from build123d import *

# Parameters (mm, degrees)
F1_DEPTH = 90
F2_R     = 10
F3_DEPTH = 300
F4_R     = 5
F5_DEPTH = 104.001


with BuildPart() as f1:
    # F0 (on Front) → F1 (new body)
    with BuildSketch(Plane.XZ):
        Polygon((50, 0), (0, 0), (-50, 0), (-50, 150), (-52, 150), (-52, -2), (52, -2), (52, 150), (50, 150), align=None)
    extrude(amount=F1_DEPTH)

    # F2 (on face) → F3 (join)
    with BuildSketch(Plane(origin=(0, 0, -2), x_dir=(1, 0, 0), z_dir=(0, 0, -1))):
        with Locations((0, 45)):
            Circle(F2_R)
    extrude(amount=F3_DEPTH)

    # F4 (on face) → F5 (cut, through all)
    with BuildSketch(Plane(origin=(-52, 0, 0), x_dir=(0, -1, 0), z_dir=(-1, 0, 0))):
        with Locations((45, 100)):
            Circle(F4_R)
        with Locations((45, 50)):
            Circle(F4_R)
    extrude(amount=-F5_DEPTH, mode=Mode.SUBTRACT)


solid = f1.part
Can you work these out from the model? Positions are in its coordinate system, mm. A direction names the side the tool comes from. Coordinates: 2 decimals unless noted, no trailing zeros. Write each loop counter-clockwise with the first axis right and the second up, starting at its lowest first coordinate (ties: lowest second). Pieces come first, ordered by that corner, then holes. Notation, with made-up numbers: (-37.75, 3.25) -> (8.25, 3.25) arc R20 cw to (8.25, 27.25) -> close; hole circle Ø5 at (52.5, -8.5). An arc over 180 degrees is marked (long way). Write each question's results on one line, items separated by ' | '. Start each with the question number.
Item 1: If we section it at B-B, the plane y = -15.5: Write out the boundary of the cut face in (x, z), and give its area (3 significant figures).
Item 2: If we section it at D-D, the plane z = -119: Write out the boundary of the cut face in (x, y), and give its area (3 significant figures).
Item 3: If we section it at A-A, the plane z = 50: Write out the boundary of the cut face in (x, y), and give its area (3 significant figures).
Item 4: Thinking about a two-plate mould opening in X: for faces 1 (the flat face through (-50.3, 0, 74.4)), 2 (the cylindrical face through (-2.17, -35.24, -149.9)), 3 (the flat face through (1, -44, 0)), 4 (the flat face through (-50, -44, 74)), which applies, released by +X, released by -X, zero draft, split by the parting line, or undercut?
Item 5: I'm going to push flat-ended pins straight in: P1, Ø11.5, axis at y = -45, z = 100, coming from the -X side; P2, Ø1.5, axis at x = -9.5, z = -116, coming from the -Y side; P3, Ø6, axis at x = 31.5, y = -62, coming from the +Z side; P4, Ø5, axis at y = -46.5, z = -154.5, coming from the -X side. Where does each tip first touch, or does it pass through?
Item 6: Please list where these lines run through material, in increasing order: probe 1 along Z at (x, y) = (50.5, -45); probe 2 along X at (y, z) = (-32, 126.5); probe 3 along Z at (x, y) = (-22, -53).
Item 7: On a 3-axis mill with a long thin cutter (end or side, diameter ignored), from which of +Z, -Z, +X, -X, +Y, -Y can I reach the whole of each face in a straight line? I mean faces 5 (the flat face through (-50.3, -90, 74.4)), 6 (the flat face through (50, -44, 76)). Say none if no direction works.
Item 8: If we section it at C-C, the plane x = 0: Write out the boundary of the cut face in (y, z), and give its area (3 significant figures).
Answer block:
1) outline: (-52, -2) -> (52, -2) -> (52, 150) -> (50, 150) -> (50, 0) -> (-50, 0) -> (-50, 150) -> (-52, 150) -> close | area: 808 mm²
2) outline: circle Ø20 at (0, -45) | area: 314 mm²
3) outline: (-52, -90) -> (-50, -90) -> (-50, -50) -> (-52, -50) -> close; (-52, -40) -> (-50, -40) -> (-50, 0) -> (-52, 0) -> close; (50, -90) -> (52, -90) -> (52, -50) -> (50, -50) -> close; (50, -40) -> (52, -40) -> (52, 0) -> (50, 0) -> close | area: 320 mm²
4) face 1: zero draft | face 2: split by the parting line | face 3: undercut | face 4: undercut
5) P1: x = -52 | P2: y = -49.84 | P3: z = 0 | P4: x = -10
6) probe 1: -2 to 45, 55 to 95, 105 to 150 | probe 2: -52 to -50, 50 to 52 | probe 3: -2 to 0
7) face 5: +Z, -Z, +X, -X, -Y | face 6: +Z, +Y, -Y
8) outline: (-90, -2) -> (-55, -2) -> (-55, -302) -> (-35, -302) -> (-35, -2) -> (0, -2) -> (0, 0) -> (-90, 0) -> close | area: 6,180 mm²
